The listing builds one solid part. Answer for the finished solid, in the listing's coordinates (mm). Face numbers are marked on the shaded views. A direction names the side the tool comes from. Coordinates: 2 decimals unless noted, no trailing zeros. Write each loop counter-clockwise with the first axis right and the second up, starting at its lowest first coordinate (ties: lowest second). Pieces come first, ordered by that corner, then holes.
(1) Straight lines are drawn through the part: line 1 (Z direction, x = 8.5, y = -107); line 2 (Z direction, x = 31, y = -110.5); line 3 (X direction, y = -114.25, z = 11.25). For each, find the intervals that lie inside material, in ascending order.
(2) The part is cut by section A-A on x = 28. Determine the outline of the cut face in (y, z).
(3) Which of the six approach directions +Z, -Z, +X, -X, +Y, -Y give full straight-line access (tool end or side, diameter ignored) to the marked faces 1 and 2?
(4) Given P1, Ø4, axis at x = 22.5, y = -110, coming from the +Z side; P2, Ø0.8, axis at x = 36, y = -116, coming from the +Z side; P3, Ø2, axis at y = -111.5, z = 11, coming from the -X side, each flat-ended and moving along its own axis, determine where each tip first touches the part or whether it passes through.
(5) The part is cut by section C-C on z = 10.5. Determine the outline of the cut face in (x, y), plus the area to 3 significant figures.
(6) The part is cut by section D-D on y = -111. Determine the outline of the cut face in (x, z), plus the area to 3 significant figures.
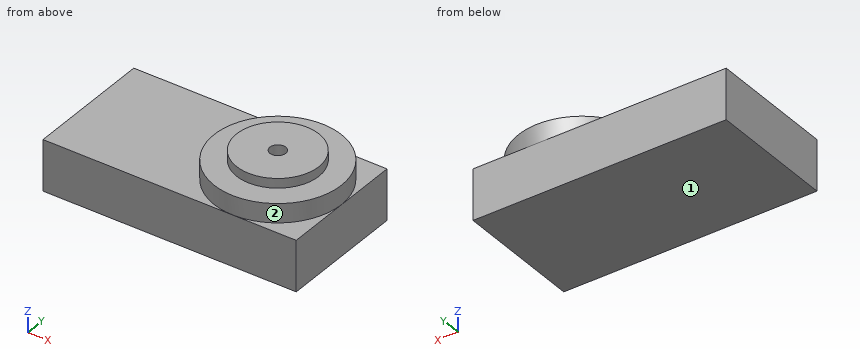
from build123d import *

# Parameters (mm, degrees)
SKETCH1_W           = 39.958127878
SKETCH1_H           = 20.143584626
BOSS_EXTRUDE1_DEPTH = 8
SKETCH2_R           = 10.049780621
BOSS_EXTRUDE2_DEPTH = 3
SKETCH3_R           = 6.5
BOSS_EXTRUDE3_DEPTH = 1.5
SKETCH4_R           = 1.25
CUT_EXTRUDE1_DEPTH  = 5


with BuildPart() as part:
    # Sketch1 → Boss-Extrude1 (new body)
    with BuildSketch(Plane.XY):
        with Locations((25.688484617, -116.024886289)):
            Rectangle(SKETCH1_W, SKETCH1_H)
    extrude(amount=BOSS_EXTRUDE1_DEPTH)

    # Sketch2 → Boss-Extrude2 (add)
    with BuildSketch(Plane.XY.offset(8)):
        with Locations((35.597548556, -116.024886289)):
            Circle(SKETCH2_R)
    extrude(amount=BOSS_EXTRUDE2_DEPTH)

    # Sketch3 → Boss-Extrude3 (add)
    with BuildSketch(Plane.XY.offset(11)):
        with Locations((35.597548556, -116.024886289)):
            Circle(SKETCH3_R)
    extrude(amount=BOSS_EXTRUDE3_DEPTH)

    # Sketch4 → Cut-Extrude1 (cut)
    with BuildSketch(Plane.XY.offset(12.5)):
        with Locations((35.597548556, -116.024886289)):
            Circle(SKETCH4_R)
    extrude(amount=-CUT_EXTRUDE1_DEPTH, mode=Mode.SUBTRACT)


solid = part.part
Model answer:
1. line 1: z = 0 to 8
1. line 2: z = 0 to 11
1. line 3: x = 29.34 to 41.85
2. outline: (-126.1, 0) - (-105.95, 0) - (-105.95, 8) - (-109.45, 8) - (-109.45, 11) - (-122.6, 11) - (-122.6, 8) - (-126.1, 8) - close
3. face 1: -Z, +X, -X, +Y, -Y
3. face 2: +Z
4. P1: stops at z = 8
4. P2: stops at z = 7.5
4. P3: stops at x = 26.19
5. outline: circle Ø20.1 at (35.6, -116.02); hole circle Ø2.5 at (35.6, -116.02)
5. area: 312 mm2
6. outline: (5.71, 0) - (45.67, 0) - (45.67, 8) - (44.3, 8) - (44.3, 11) - (39.72, 11) - (39.72, 12.5) - (31.47, 12.5) - (31.47, 11) - (26.89, 11) - (26.89, 8) - (5.71, 8) - close
6. area: 384 mm2
